Part print with two shaded views. Sizes in mm from the minimum x, y, z corner. A direction names the side the tool comes from. Coordinates: 2 decimals unless noted, no trailing zeros. Write each loop counter-clockwise with the first axis right and the second up, starting at its lowest first coordinate (ties: lowest second). Pieces come first, ordered by that corner, then holes. Notation, with made-up numbers: (18.5, 45) - (59.5, 45) arc R19 cw to (59.5, 68) - close; hole circle Ø10 at (58.25, -21.75). An arc over 180 degrees is marked (long way). Answer in a Markdown table with one row per item. Add a question column.
Q1. Drill centre lines: line 1 along Z through (x, y) = (93, 3); line 2 along Y through (x, z) = (105, 37); line 3 along Y through (x, z) = (101, 6). Where is each one in solid material? Low to high. Write a range as from..to.
Q2. Band-saw the part on D-D (x = 75). List the corners of the cut face in (y, z), and give its area (3 significant figures).
Q3. Band-saw the part on C-C (z = 6). List the corners of the cut face in (x, y).
Q4. Pin check, flat tips, straight feed: pin 1 (18 mm diameter, centred on x = 105, y = 25, fed in from -Z); pin 2 (3 mm diameter, centred on y = 38, z = 23.5, fed in from +X); pin 3 (3 mm diameter, centred on y = 21.5, z = 31, fed in from -X). Stop position of each tip, or through.
Q5. Band-saw the part on A-A (y = 25). List the corners of the cut face in (x, z).
Q6. Band-saw the part on B-B (x = 105). List the corners of the cut face in (y, z).
Q7. 3-axis set-ups, long thin cutter, end or side, ignore diameter. For the marked faces 4 and 5: which of +Z, -Z, +X, -X, +Y, -Y reach the whole face in a straight line?
Q8. Two-plate mould, pull along Y, no slides. Class the marked faces 1, 2 and 3: +Y half, -Y half, draft (parallel to the pull), parting line (faces both ways), or undercut.
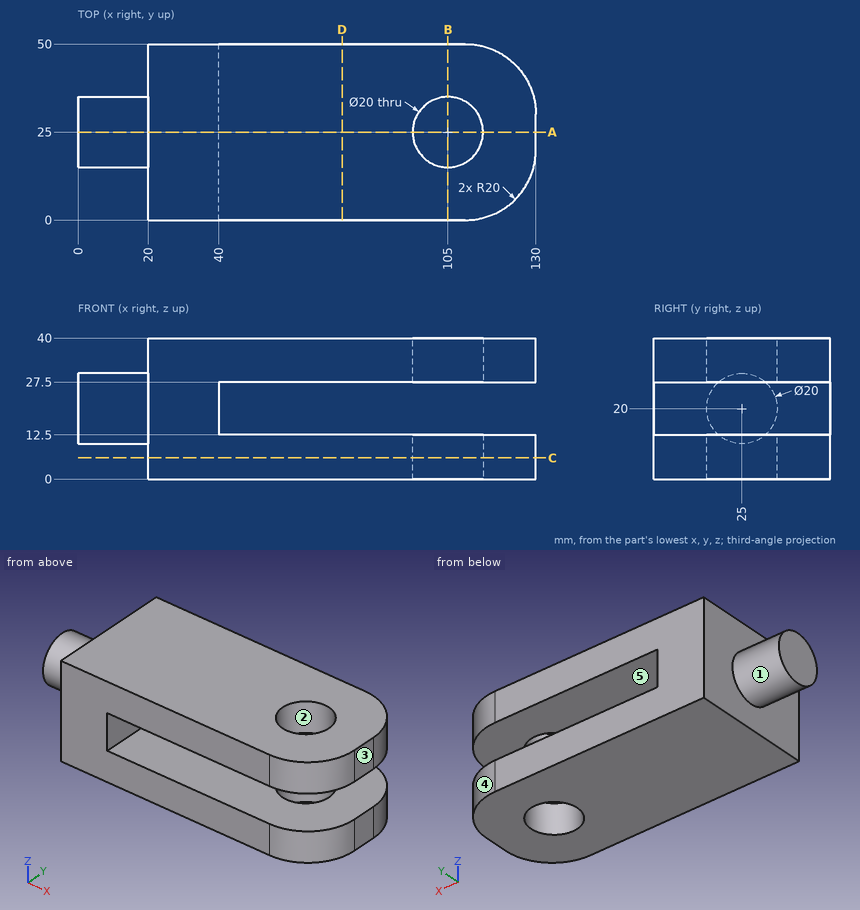
Checked values:
| question | item | result |
|---|---|---|
| 1 | line 1 | z = 0..12.5, 27.5..40 |
| 1 | line 2 | y = 0..15, 35..50 |
| 1 | line 3 | y = 0..15.83, 34.17..50 |
| 2 | outline | (0, 0) - (50, 0) - (50, 12.5) - (0, 12.5) - close; (0, 27.5) - (50, 27.5) - (50, 40) - (0, 40) - close |
| 2 | area | 1,250 mm² |
| 3 | outline | (20, 0) - (110, 0) arc R20 ccw to (130, 20) - (130, 30) arc R20 ccw to (110, 50) - (20, 50) - close; hole circle Ø20 at (105, 25) |
| 4 | pin 1 | passes through |
| 4 | pin 2 | stops at x = 40 |
| 4 | pin 3 | stops at x = 20 |
| 5 | outline | (0, 10) - (20, 10) - (20, 0) - (95, 0) - (95, 12.5) - (40, 12.5) - (40, 27.5) - (95, 27.5) - (95, 40) - (20, 40) - (20, 30) - (0, 30) - close; (115, 0) - (130, 0) - (130, 12.5) - (115, 12.5) - close; (115, 27.5) - (130, 27.5) - (130, 40) - (115, 40) - close |
| 6 | outline | (0, 0) - (15, 0) - (15, 12.5) - (0, 12.5) - close; (0, 27.5) - (15, 27.5) - (15, 40) - (0, 40) - close; (35, 0) - (50, 0) - (50, 12.5) - (35, 12.5) - close; (35, 27.5) - (50, 27.5) - (50, 40) - (35, 40) - close |
| 7 | face 4 | +Z, -Z, +X, +Y |
| 7 | face 5 | +X, +Y, -Y |
| 8 | face 1 | parting line |
| 8 | face 2 | undercut |
| 8 | face 3 | draft |
